Input: dimensioned drawing with shaded views. Units: mm. Origin: part minimum x, y, z. A direction names the side the tool comes from. Give positions to 0.01 mm unless a question says otherwise; leave off trailing zeros. Loops run counter-clockwise (first coordinate to the right, second up) from the corner with the lowest first, then second, coordinate; pieces in that order, holes last. Notation, with made-up numbers: (-34.5, 41) -> (-12.5, 41) arc R34 cw to (-12.5, 74) -> close; hole circle Ø6 at (-13, 72). An arc over 180 degrees is marked (long way). Answer in a Markdown table with one row per item. Add a question column.
1) Line query: line 1 (Z direction, x = 3.5, y = 1); line 2 (Y direction, x = 8.5, z = 2.5); line 3 (Z direction, x = 3.5, y = 4). Output: solid intervals per line, ascending. Write a range as from..to.
2) Section query B-B (x = 5). Return the cut outline in (y, z).
3) Access query for the marked faces 4, 5 and 6. Directions: +Z, -Z, +X, -X, +Y, -Y. A direction counts if a zero-diameter tool reaches every point of the face in a straight line with its end or side. Return the directions, or none.
4) Draft query along Y for the marked faces 1, 2 and 3. Return one class per face: +Y half, -Y half, draft (parallel to the pull), parting line (faces both ways), or undercut.
5) Section query C-C (y = 8.75). Return the cut outline in (x, z).
6) Section query A-A (z = 2.75). Return the cut outline in (x, y).
7) Section query D-D (x = 1). Return the cut outline in (y, z).
8) First-contact query: P1, Ø4, axis at y = 2, z = 3, coming from the +X side; P2, Ø1.5, axis at x = 5.5, z = 5.5, coming from the +Y side (1 decimal). Flat tips, straight axial feed; report the tip coordinate or a pass-through.
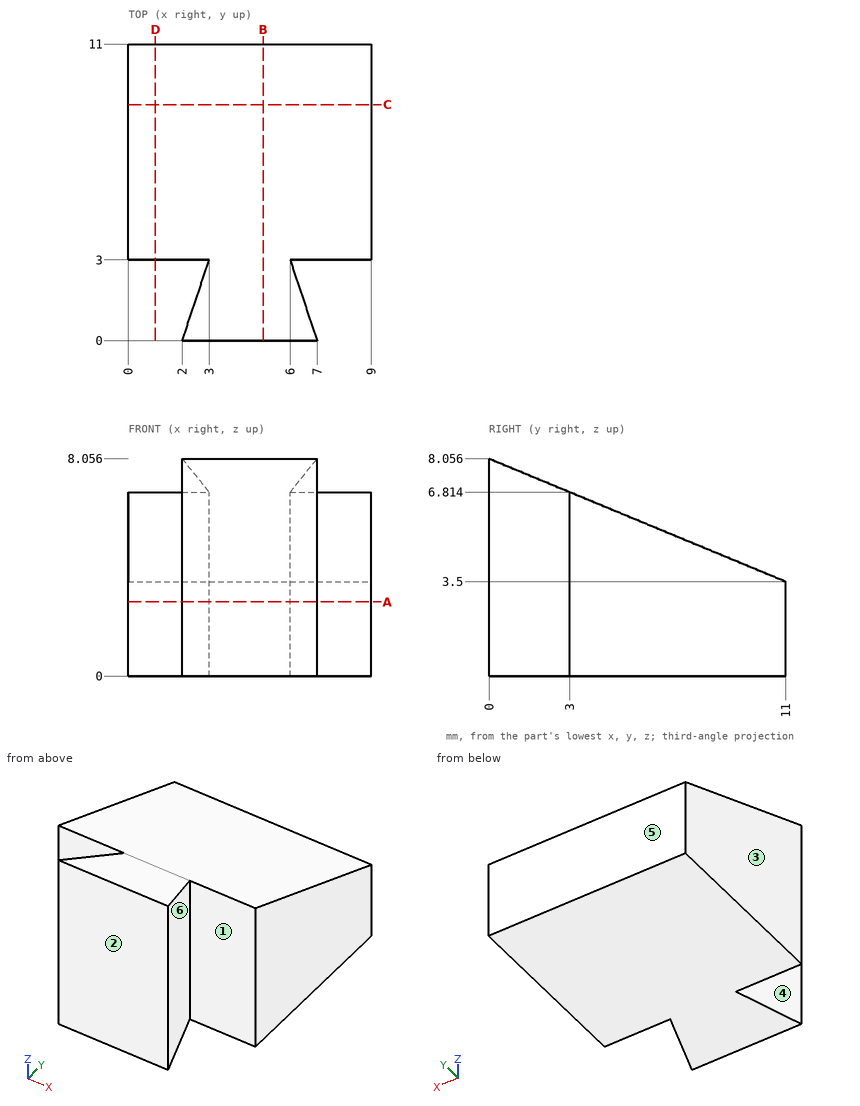
Evaluation:
| question | item | result |
|---|---|---|
| 1 | line 1 | 0..7.64 |
| 1 | line 2 | 3..11 |
| 1 | line 3 | 0..6.4 |
| 2 | outline | (0, 0) -> (11, 0) -> (11, 3.5) -> (0, 8.06) -> close |
| 3 | face 4 | +Z, -Z, -X |
| 3 | face 5 | +Z, -Z, +X, -X, +Y |
| 3 | face 6 | +Z, -Z, +X |
| 4 | face 1 | undercut |
| 4 | face 2 | -Y half |
| 4 | face 3 | draft |
| 5 | outline | (0, 0) -> (9, 0) -> (9, 4.43) -> (0, 4.43) -> close |
| 6 | outline | (0, 3) -> (3, 3) -> (2, 0) -> (7, 0) -> (6, 3) -> (9, 3) -> (9, 11) -> (0, 11) -> close |
| 7 | outline | (3, 0) -> (11, 0) -> (11, 3.5) -> (3, 6.81) -> close |
| 8 | P1 | x = 9 |
| 8 | P2 | y = 8 |
